Verification items for the finished model (mm, model axes). Coordinates: 2 decimals unless noted, no trailing zeros. Order: outer loops, then holes, each group sorted by start corner. A loop starts at its lowest first (then second) coordinate and runs counter-clockwise, first axis right, second up. Notation, with made-up numbers: M -21.75,36.5 L -13.75,36.5 A17 ccw -13.75,50.5 Z; hole C 78,85 d9. An arc over 180 degrees is marked long. Return JSON: item names as keys, results as strings.
```python
from build123d import *

# Parameters (mm, degrees)
SKETCH1_W           = 20
SKETCH1_H           = 20
SKETCH1_R           = 8
BOSS_EXTRUDE1_DEPTH = 4
SKETCH3_R           = 1
CUT_EXTRUDE1_DEPTH  = 20


with BuildPart() as part:
    # Sketch1 → Boss-Extrude1 (new body)
    with BuildSketch(Plane.XY):
        Rectangle(SKETCH1_W, SKETCH1_H)
        Circle(SKETCH1_R, mode=Mode.SUBTRACT)
    extrude(amount=BOSS_EXTRUDE1_DEPTH)

    # Sketch3 → Cut-Extrude1 (cut)
    with BuildSketch(Plane(origin=(0, 10, 0), x_dir=(1, 0, 0), z_dir=(0, 1, 0))):
        with Locations(Location((0, -2, 0), (0, 0, 270))):
            Circle(SKETCH3_R)
    extrude(amount=-CUT_EXTRUDE1_DEPTH, mode=Mode.SUBTRACT)


solid = part.part
```
Q1. Cross-section at C-C, the plane y = 0. Record the boundary of the cut face in (x, z), and give its area (3 significant figures).
Values:
{"outline": "M -10,0 L -8,0 L -8,4 L -10,4 Z; M 8,0 L 10,0 L 10,4 L 8,4 Z", "area": "16.0 mm^2"}
Q2. Cross-section at D-D, the plane y = 8.75. Record the boundary of the cut face in (x, z), and give its area (3 significant figures).
Values:
{"outline": "M -10,0 L 10,0 L 10,4 L -10,4 Z; hole C 0,2 d2", "area": "76.9 mm^2"}
Q3. Go/stop test with a flat-tipped pin: pin 1 (6 mm diameter, centred on x = -6, y = 2.5, fed in from -Z). Record where the tip stops, or that it passes through.
Values:
{"pin 1": "z = 0"}
Q4. Material ranges on line 1 along X through (y, z) = (-9.05, 2); line 2 along Z through (x, y) = (0, 9.3); line 3 along Y through (x, z) = (7, 1.8), recorded low to high.
Values:
{"line 1": "-10 to -1, 1 to 10", "line 2": "0 to 1, 3 to 4", "line 3": "-10 to -3.87, 3.87 to 10"}
Q5. Draft check along Y on faces 1 (the face through (-0.1, 10, 3.3)), 2 (the face through (-1.73, -7.81, 1.97)), 3 (the face through (-0.6, 9, 1.2)). Enter one of: pulls with the +Y half, pulls with the -Y half, needs draft (parallel to the pull), parting line crosses it, or undercut.
Values:
{"face 1": "pulls with the +Y half", "face 2": "undercut", "face 3": "needs draft"}
Q6. Cross-section at A-A, the plane z = 2. Record the boundary of the cut face in (x, y).
Values:
{"outline": "M -10,-10 L -1,-10 L -1,-7.94 A8 cw -1,7.94 L -1,10 L -10,10 Z; M 1,-10 L 10,-10 L 10,10 L 1,10 L 1,7.94 A8 cw 1,-7.94 Z"}
Q7. Cross-section at B-B, the plane x = 0. Record the boundary of the cut face in (y, z), and give its area (3 significant figures).
Values:
{"outline": "M -10,0 L -8,0 L -8,1 L -10,1 Z; M -10,3 L -8,3 L -8,4 L -10,4 Z; M 8,0 L 10,0 L 10,1 L 8,1 Z; M 8,3 L 10,3 L 10,4 L 8,4 Z", "area": "8.00 mm^2"}
